Read the model definition and answer for the solid it produces. Units are mm, in the model's axes. Face numbers are marked on the shaded views. A direction names the side the tool comes from. Give positions to 0.01 mm unless a question says otherwise; leave off trailing zeros. Loops run counter-clockwise (first coordinate to the right, second up) from the corner with the lowest first, then second, coordinate; pieces in that order, holes last.
(1) Find section D-D, the plane z = 52.5. Write down the section's boundary in (x, y), then the cut area to 3 significant figures.
(2) Straight lines are drawn through the part: probe 1 along X at (y, z) = (10.5, 63); probe 2 along Y at (x, z) = (30, 39.5); probe 3 along X at (y, z) = (72, 31.5) (3 decimals). For each, find the intervals that lie inside material, in ascending order.
(3) Which of the six approach directions +Z, -Z, +X, -X, +Y, -Y give full straight-line access (tool end or side, diameter ignored) to the marked faces 1, 2 and 3?
(4) Find section C-C, the plane z = 23.5. Write down the section's boundary in (x, y).
(5) Each of these flat-tipped pins is pushed along its axis until it touches: P1, Ø18, axis at x = 11.5, z = 23, coming from the -Y side; P2, Ø3, axis at y = 41, z = 27.5, coming from the -X side; P3, Ø6, axis at x = -34.5, y = 76.5, coming from the +Z side; P4, Ø15.5, axis at x = 12, z = 40.5, coming from the -Y side. Where does it stop, or does it pass through?
(6) Find section A-A, the plane y = 18. Write down the section's boundary in (x, z).
(7) Determine the mould class of the marked faces 4, 5, 6 and 7 for opening direction X: pulls with the +X half, pulls with the -X half, needs draft (parallel to the pull), parting line crosses it, or undercut.
(8) Find section B-B, the plane x = -39. Write down the section's boundary in (y, z), then the cut area to 3 significant figures.
```python
from build123d import *

# Parameters (mm, degrees)
BOSS_EXTRUDE1_DEPTH             = 70
CUT_EXTRUDE1_DEPTH              = 200.200903612
FILLET1_R                       = 25
BOSS_EXTRUDE2_REACH             = 139.891
SKETCH3_W                       = 3
SKETCH3_H                       = 8
BOSS_EXTRUDE2_DIRECTION_2_REACH = 139.891
FILLET2_R                       = 10


with BuildPart() as part:
    # Sketch1 → Boss-Extrude1 (new body)
    with BuildSketch(Plane.XY):
        with BuildLine():
            Line((-83, 5), (-83, 65))
            ThreePointArc((-83, 65), (-77.142135624, 79.142135624), (-63, 85))
            Line((-63, 85), (63, 85))
            ThreePointArc((63, 85), (77.142135624, 79.142135624), (83, 65))
            Line((83, 65), (83, 5))
            Line((83, 5), (80, 5))
            Line((80, 5), (80, 65))
            ThreePointArc((80, 65), (75.02081528, 77.02081528), (63, 82))
            Line((63, 82), (-63, 82))
            ThreePointArc((-63, 82), (-75.02081528, 77.02081528), (-80, 65))
            Line((-80, 65), (-80, 5))
            Line((-80, 5), (-83, 5))
        make_face()
    extrude(amount=BOSS_EXTRUDE1_DEPTH)

    # Sketch2 → Cut-Extrude1 (cut, through all)
    with BuildSketch(Plane.ZY.offset(83)):
        Polygon((49.016155383, 85), (70, 40), (70, 85), align=None)
        Polygon((10.397928219, 85), (35, 32.240686807), (35, 4.870884332), (0, 4.870884332), (0, 85), align=None)
    extrude(amount=-CUT_EXTRUDE1_DEPTH, mode=Mode.SUBTRACT)

    # Fillet1
    fillet1_edges = [part.edges().sort_by_distance(p)[0] for p in [
        (-81.5, 40, 70),
        (81.5, 40, 70),
        (-81.5, 32.240686807, 35),
        (81.5, 32.240686807, 35),
    ]]
    fillet(fillet1_edges, radius=FILLET1_R)

    # Sketch3 → Boss-Extrude2 (add, up to next)
    with BuildSketch(Plane(origin=(0, 0, 0), x_dir=(0, 0, -1), z_dir=(1, 0, 0)), mode=Mode.PRIVATE) as boss_extrude2_sk1:
        with Locations((-29.707041801, 81)):
            Rectangle(SKETCH3_W, SKETCH3_H)
    boss_extrude2_tool1 = extrude(boss_extrude2_sk1.sketch, amount=BOSS_EXTRUDE2_REACH, mode=Mode.PRIVATE) - part.part
    add(boss_extrude2_tool1.solids().sort_by_distance((0, 81, 29.707042))[0])

    # Sketch3 → Boss-Extrude2 direction 2 (add, up to next)
    with BuildSketch(Plane(origin=(0, 0, 0), x_dir=(0, 0, -1), z_dir=(1, 0, 0)), mode=Mode.PRIVATE) as boss_extrude2_direction_2_sk1:
        with Locations((-29.707041801, 81)):
            Rectangle(SKETCH3_W, SKETCH3_H)
    boss_extrude2_direction_2_tool1 = extrude(boss_extrude2_direction_2_sk1.sketch, amount=-BOSS_EXTRUDE2_DIRECTION_2_REACH, mode=Mode.PRIVATE) - part.part
    add(boss_extrude2_direction_2_tool1.solids().sort_by_distance((0, 81, 29.707042))[0])

    # Fillet2
    fillet2_edges = [part.edges().sort_by_distance(p)[0] for p in [
        (-75.041594579, 77, 29.707041801),
        (75.041594579, 77, 29.707041801),
    ]]
    fillet(fillet2_edges, radius=FILLET2_R)


solid = part.part
```
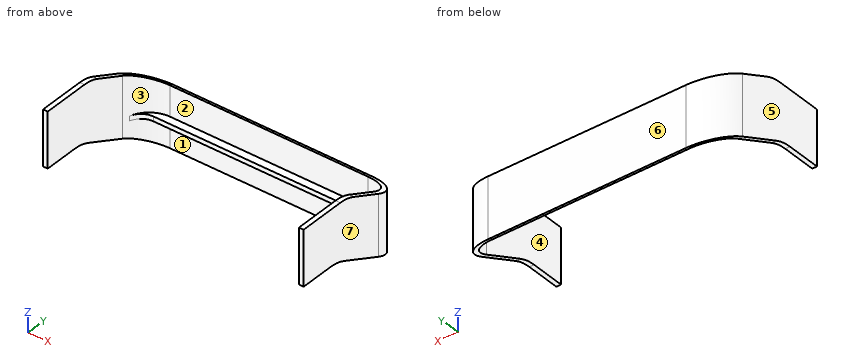
Entries:
1. outline: (-83, 5) - (-80, 5) - (-80, 65) arc R17 cw to (-74.49, 77.53) - (-78.59, 77.53) arc R20 ccw to (-83, 65) - close; (74.49, 77.53) arc R17 cw to (80, 65) - (80, 5) - (83, 5) - (83, 65) arc R20 ccw to (78.59, 77.53) - close
1. area: 443 mm2
2. probe 1: x = -83 to -80, 80 to 83
2. probe 2: y = 82 to 85
2. probe 3: x = -81.735 to -78.492, 78.492 to 81.735
3. face 1: -Z, -Y
3. face 2: +Z, -Y
3. face 3: -Y
4. outline: (-83, 56.9) - (-80, 56.9) - (-80, 65) arc R17 cw to (-63, 82) - (63, 82) arc R17 cw to (80, 65) - (80, 56.9) - (83, 56.9) - (83, 65) arc R20 ccw to (63, 85) - (-63, 85) arc R20 ccw to (-83, 65) - close
5. P1: stops at y = 77
5. P2: passes through
5. P3: stops at z = 31.21
5. P4: stops at y = 82
6. outline: (-83, 35) - (-80, 35) - (-80, 70) - (-83, 70) - close; (80, 35) - (83, 35) - (83, 70) - (80, 70) - close
7. face 4: undercut
7. face 5: pulls with the -X half
7. face 6: needs draft
7. face 7: pulls with the +X half
8. outline: (77, 28.21) - (82, 28.21) - (82, 11.8) - (85, 10.4) - (85, 49.02) - (82, 50.42) - (82, 31.21) - (77, 31.21) - close
8. area: 131 mm2
